from build123d import *

# Parameters (mm, degrees)
F0_W     = 31.8008
F0_H     = 15.875
F1_DEPTH = 9.6012
F2_R     = 2.4267031392
F3_DEPTH = 1.8796
F4_T     = -1.27
F5_R     = 2.4257
F6_DEPTH = 8.3312
F7_R     = 2.1361983008
F8_DEPTH = 8.3312


with BuildPart() as f1:
    # F0 (on Front) → F1 (new body)
    with BuildSketch(Plane.XZ):
        with Locations((-1.5301071107, -3.5654834016)):
            Rectangle(F0_W, F0_H)
    extrude(amount=F1_DEPTH)

    # F2 (on face) → F3 (join)
    with BuildSketch(Plane.XZ.offset(9.6012)):
        with Locations((10.6989897501, -7.8316802624)):
            Circle(F2_R)
        with Locations((2.9773897501, -7.8316802624)):
            Circle(F2_R)
        with Locations((-4.7442102499, -7.8316802624)):
            Circle(F2_R)
        with Locations((-12.4658102499, -7.8316802624)):
            Circle(F2_R)
        with Locations((2.9773897501, 0.7007134592)):
            Circle(F2_R)
        with Locations((-4.7442102499, 0.7007134592)):
            Circle(F2_R)
        with Locations((-12.4658102499, 0.7007134592)):
            Circle(F2_R)
        with Locations((10.6989897501, 0.7007134592)):
            Circle(F2_R)
    extrude(amount=F3_DEPTH)

    # F4
    f4_openings = [f1.faces().sort_by_distance(p)[0] for p in [
        (-1.530107, 0, -3.565483),
    ]]
    offset(amount=F4_T, openings=f4_openings, kind=Kind.INTERSECTION)

    # F5 (on face) → F6 (join, through all)
    with BuildSketch(Plane(origin=(0, -8.3312, 0), x_dir=(-1, 0, 0), z_dir=(0, 1, 0))):
        with Locations((1.5301071107, -3.5654834016)):
            Circle(F5_R)
        with Locations((8.8453071107, -3.5654834016)):
            Circle(F5_R)
        with Locations((-5.7850928893, -3.5654834016)):
            Circle(F5_R)
    extrude(amount=F6_DEPTH)

    # F7 (on face) → F8 (cut, through all)
    with BuildSketch(Plane(origin=(0, 0, 0), x_dir=(-1, 0, 0), z_dir=(0, 1, 0))):
        with Locations((-5.7850928893, -3.5654834016)):
            Circle(F7_R)
        with Locations((1.5387871107, -3.5654834016)):
            Circle(F7_R)
        with Locations((8.8626671107, -3.5654834016)):
            Circle(F7_R)
    extrude(amount=-F8_DEPTH, mode=Mode.SUBTRACT)


solid = f1.part
Input: part model. Units: mm. Frame: model coordinates. A direction names the side the tool comes from. Coordinates: 2 decimals unless noted, no trailing zeros. Loops run counter-clockwise (first coordinate to the right, second up) from the corner with the lowest first, then second, coordinate; pieces in that order, holes last. Notation, with made-up numbers: (6, -5) -> (24, -5) arc R13 cw to (24, 15) -> close; hole circle Ø7 at (-38, 59). An arc over 180 degrees is marked (long way). Write each question's results on one line, items separated by ' | '. Start each with the question number.
Q1. Pin query (flat end, axial travel): pin 1 (0.7 mm diameter, centred on x = -13, z = 0, fed in from +Y); pin 2 (3.5 mm diameter, centred on x = 5.79, z = -3.57, fed in from -Y); pin 3 (1.2 mm diameter, centred on x = -12.5, z = -8, fed in from +Y). Return the tip coordinate at first contact, or that it passes through.
Q2. Section B-B, the plane y = -6. Return the cut outline in (x, z), plus the area to 3 significant figures.
Q3. Section A-A, the plane y = -10.75. Return the cut outline in (x, z), plus the area to 3 significant figures.
Q4. Pull-direction query (Z, two-part tool) for faces 3 (the cylindrical face through (-1.08, -4.11, -5.65)), 4 (the flat face through (-5, -11.481, 1)), 5 (the cylindrical face through (5.3, -10.5, 1.4)); classes: released by +Z, released by -Z, zero draft, split by the parting line, or undercut.
Q5. Reachability of faces 1 (the cylindrical face through (13.014, -10.528, 1.43)), 2 (the cylindrical face through (4.046, -9.258, 0.258)) from +Z, -Z, +X, -X, +Y, -Y: full face, straight path, thin tool, end or side. Return the list, or none.
Q6. Section D-D, the plane x = 6. Return the cut outline in (y, z), plus the area to 3 significant figures.
Q7. Ray query, line 1 (Z direction, x = -9, y = -6.75); line 2 (X direction, y = -3, z = 1.75); line 3 (Z direction, x = 9.5, y = -7.5). Return the intervals inside material, ascending. Write a range as from..to.
Found:
1) pin 1: y = -8.33 | pin 2: y = -9.6 | pin 3: y = -10.21
2) outline: (-17.43, -11.5) -> (14.37, -11.5) -> (14.37, 4.37) -> (-17.43, 4.37) -> close; circle Ø4.85 at (-8.85, -3.57); circle Ø4.85 at (-1.53, -3.57); circle Ø4.85 at (5.79, -3.57); hole (-16.16, -10.23) -> (13.1, -10.23) -> (13.1, 3.1) -> (-16.16, 3.1) -> close; hole circle Ø4.27 at (-8.86, -3.57); hole circle Ø4.27 at (-1.54, -3.57); hole circle Ø4.27 at (5.79, -3.57) | area: 127 mm2
3) outline: circle Ø4.85 at (-12.47, -7.83); circle Ø4.85 at (-12.47, 0.7); circle Ø4.85 at (-4.74, -7.83); circle Ø4.85 at (-4.74, 0.7); circle Ø4.85 at (2.98, -7.83); circle Ø4.85 at (2.98, 0.7); circle Ø4.85 at (10.7, -7.83); circle Ø4.85 at (10.7, 0.7) | area: 148 mm2
4) face 3: undercut | face 4: zero draft | face 5: undercut
5) face 1: -Y | face 2: +Y
6) outline: (-9.6, -11.5) -> (0, -11.5) -> (0, -10.23) -> (-8.33, -10.23) -> (-8.33, -5.98) -> (0, -5.98) -> (0, -5.69) -> (-8.33, -5.69) -> (-8.33, -1.44) -> (0, -1.44) -> (0, -1.15) -> (-8.33, -1.15) -> (-8.33, 3.1) -> (0, 3.1) -> (0, 4.37) -> (-9.6, 4.37) -> close | area: 46.2 mm2
7) line 1: -11.5..-10.23, -5.99..-5.7, -1.43..-1.14, 3.1..4.37 | line 2: -17.43..-16.16, 13.1..14.37 | line 3: -11.5..-10.23, 3.1..4.37
